from build123d import *

# Parameters (mm, degrees)
SKETCH1_W           = 50
SKETCH1_H           = 40
SKETCH1_R           = 1.5
BOSS_EXTRUDE1_DEPTH = 10
CUT_EXTRUDE2_DEPTH  = 50
SKETCH4_W           = 39.996802558
SKETCH4_H           = 5
BOSS_EXTRUDE2_DEPTH = 20
SKETCH5_W           = 5
SKETCH5_H           = 39.996802558
BOSS_EXTRUDE3_DEPTH = 50
SKETCH6_W           = 39.996802558
SKETCH6_H           = 5
BOSS_EXTRUDE4_DEPTH = 15
SKETCH9_R           = 2
CUT_EXTRUDE6_DEPTH  = 5


with BuildPart() as part:
    # Sketch1 → Boss-Extrude1 (new body)
    with BuildSketch(Plane(origin=(0, 0, 0), x_dir=(1, 0, 0), z_dir=(0, 1, 0))):
        Rectangle(SKETCH1_W, SKETCH1_H)
        with Locations(Location((5, 0, 0), (0, 0, 270))):
            Circle(SKETCH1_R, mode=Mode.SUBTRACT)
        with Locations(Location((-5, 0, 0), (0, 0, 90))):
            Circle(SKETCH1_R, mode=Mode.SUBTRACT)
    extrude(amount=BOSS_EXTRUDE1_DEPTH)

    # Sketch3 → Cut-Extrude2 (cut)
    with BuildSketch(Plane.ZY.offset(25)):
        Polygon((-20, 10), (20, 5), (20, 10), align=None)
        Polygon((20, 0), (-20, 5), (-20, 0), align=None)
    extrude(amount=-CUT_EXTRUDE2_DEPTH, mode=Mode.SUBTRACT)

    # Sketch4 → Boss-Extrude2 (add)
    with BuildSketch(Plane.ZY.offset(25)):
        with Locations((0.001598721, 2.5)):
            Rectangle(SKETCH4_W, SKETCH4_H)
    boss_extrude2 = extrude(amount=BOSS_EXTRUDE2_DEPTH)

    # Sketch5 → Boss-Extrude3 (add)
    with BuildSketch(Plane.XZ):
        with Locations((-42.5, 0.001598721)):
            Rectangle(SKETCH5_W, SKETCH5_H)
    boss_extrude3 = extrude(amount=BOSS_EXTRUDE3_DEPTH)

    # Sketch6 → Boss-Extrude4 (add)
    with BuildSketch(Plane.ZY.offset(45)):
        with Locations((0.001598721, -47.5)):
            Rectangle(SKETCH6_W, SKETCH6_H)
    boss_extrude4 = extrude(amount=BOSS_EXTRUDE4_DEPTH)

    # Sketch9 → Cut-Extrude6 (cut)
    with BuildSketch(Plane(origin=(0, -45, 0), x_dir=(1, 0, 0), z_dir=(0, 1, 0))):
        with Locations(Location((-52.5, -0.001598721, 0), (0, 0, 270))):
            Circle(SKETCH9_R)
    cut_extrude6 = extrude(amount=-CUT_EXTRUDE6_DEPTH, mode=Mode.SUBTRACT)

    # Mirror3: Boss-Extrude2, Boss-Extrude3, Boss-Extrude4, Cut-Extrude6 across plane
    add(boss_extrude2.mirror(Plane(origin=(0, 0, 0), x_dir=(0, 0, 1), z_dir=(1, 0, 0))))
    add(boss_extrude3.mirror(Plane(origin=(0, 0, 0), x_dir=(0, 0, 1), z_dir=(1, 0, 0))))
    add(boss_extrude4.mirror(Plane(origin=(0, 0, 0), x_dir=(0, 0, 1), z_dir=(1, 0, 0))))
    add(cut_extrude6.mirror(Plane(origin=(0, 0, 0), x_dir=(0, 0, 1), z_dir=(1, 0, 0))), mode=Mode.SUBTRACT)


solid = part.part
The listing builds one solid part. Answer for the finished solid, in the listing's coordinates (mm). A direction names the side the tool comes from. Coordinates: 2 decimals unless noted, no trailing zeros. Write each loop counter-clockwise with the first axis right and the second up, starting at its lowest first coordinate (ties: lowest second). Pieces come first, ordered by that corner, then holes. Notation, with made-up numbers: (-14, -7.5) - (35, -7.5) arc R11 ccw to (35, -2.5) - close; hole circle Ø8 at (68, -29). An arc over 180 degrees is marked (long way). Return JSON: item names as keys, results as strings.
1. The part is cut by section C-C on x = 52.5. Determine the outline of the cut face in (y, z), then the cut area to 3 significant figures.
Final values:
{"outline": "(-50, -20) - (-45, -20) - (-45, -2) - (-50, -2) - close; (-50, 2) - (-45, 2) - (-45, 20) - (-50, 20) - close", "area": "180 mm^2"}
2. The part is cut by section D-D on x = -42. Determine the outline of the cut face in (y, z).
Final values:
{"outline": "(-50, -20) - (5, -20) - (5, 20) - (-50, 20) - close"}
3. For a pull along Z with two mould halves and no side action, classify faces 1 (the face through (-0.35, 7.535, -0.28)), 2 (the face through (-54.274, -47.465, 0.924)), 3 (the face through (-25, 1, -9)) as +Z half, -Z half, draft (parallel to the pull), parting line (faces both ways), or undercut.
Final values:
{"face 1": "+Z half", "face 2": "undercut", "face 3": "draft"}
4. Consider line 1 along X through (y, z) = (3.65, 0); line 2 along X through (y, z) = (-15, -14.5); line 3 along X through (y, z) = (5.4, 0). Determine where each line is inside the solid, lowest interval first.
Final values:
{"line 1": "-45 to -6.5, -3.5 to 3.5, 6.5 to 45", "line 2": "-45 to -40, 40 to 45", "line 3": "-25 to -6.5, -3.5 to 3.5, 6.5 to 25"}
5. Each of these flat-tipped pins is pushed along its axis until it touches: pin 1 Ø4 at (y, z) = (8, 4.5) entering from +X; pin 2 Ø5 at (x, z) = (-45, -3.5) entering from +Y; pin 3 Ø20 at (y, z) = (-26, -9) entering from +X; pin 4 Ø2.5 at (x, z) = (-5, 0) entering from +Y. Where does it stop, or does it pass through?
Final values:
{"pin 1": "x = 25", "pin 2": "y = 5", "pin 3": "x = 45", "pin 4": "through"}
6. The part is cut by section A-A on y = -37.5. Determine the outline of the cut face in (x, z), then the cut area to 3 significant figures.
Final values:
{"outline": "(-45, -20) - (-40, -20) - (-40, 20) - (-45, 20) - close; (40, -20) - (45, -20) - (45, 20) - (40, 20) - close", "area": "400 mm^2"}
7. Which of the six approach directions +Z, -Z, +X, -X, +Y, -Y give full straight-line access (tool end or side, diameter ignored) to faces 4 (the face through (-49, -45, 0)), 5 (the face through (-0.35, 2.465, 0.28)), 6 (the face through (35, 5, 0)), 7 (the face through (-40, -25, 0))?
Final values:
{"face 4": "+Z, -Z, -X, +Y", "face 5": "-Z, -Y", "face 6": "+Z, -Z, +X, +Y", "face 7": "+Z, -Z, -Y"}
8. The part is cut by section B-B on z = -4. Determine the outline of the cut face in (x, y).
Final values:
{"outline": "(-60, -50) - (-40, -50) - (-40, 0) - (-25, 0) - (-25, 3) - (25, 3) - (25, 0) - (40, 0) - (40, -50) - (60, -50) - (60, -45) - (45, -45) - (45, 5) - (25, 5) - (25, 8) - (-25, 8) - (-25, 5) - (-45, 5) - (-45, -45) - (-60, -45) - close"}
